```python
from build123d import *

# Parameters (mm, degrees)
F1_DEPTH  = 16
F2_W      = 70
F2_H      = 3
F3_DEPTH  = 2
F4_W      = 50
F4_H      = 14
F5_DEPTH  = 2
F6_R      = 1
F9_DEPTH  = 2
F11_DEPTH = 38.001
F13_D     = 4
F14_R     = 3
F14_R_2   = 2
F15_DEPTH = 5
F16_R     = 3


# Not quite as in the source:
# - a pattern or mirror of a feature is missing from the dataset's text; its kind, count and spacing are read off the source's solid


with BuildPart() as f1:
    # F0 (on Front) → F1 (new body)
    with BuildSketch(Plane.XZ):
        with BuildLine():
            Line((94, 11), (0, 11))
            ThreePointArc((0, 11), (-11, 0), (0, -11))
            Line((0, -11), (19, -11))
            ThreePointArc((19, -11), (21.7681124643, -11.8361612201), (23.6103896104, -14.064978646))
            ThreePointArc((23.6103896104, -14.064978646), (47.8977113224, -44.6078392712), (84.5520957277, -57.9942665386))
            ThreePointArc((84.5520957277, -57.9942665386), (89.5187953856, -59.3173941728), (93.6732506492, -62.3438233708))
            Line((93.6732506492, -62.3438233708), (95.1549842887, -61))
            ThreePointArc((95.1549842887, -61), (90.3976747979, -57.5207528796), (84.7034264019, -56))
            ThreePointArc((84.7034264019, -56), (49.0672193413, -42.9854179344), (25.4545454545, -13.2909701044))
            ThreePointArc((25.4545454545, -13.2909701044), (22.87535745, -10.1706257081), (19, -9))
            Line((19, -9), (0, -9))
            ThreePointArc((0, -9), (-9, 0), (0, 9))
            Line((0, 9), (94, 9))
            Line((94, 9), (94, 11))
        make_face()
    extrude(amount=F1_DEPTH)

    # F2 (on face) → F3 (join)
    with BuildSketch(Plane.XY.offset(11)):
        with Locations((59, -17.5)):
            Rectangle(F2_W, F2_H)
    extrude(amount=-F3_DEPTH)

    # F4 (on face) → F5 (join)
    with BuildSketch(Plane.XZ.offset(19)):
        with Locations((69, 2)):
            Rectangle(F4_W, F4_H)
    extrude(amount=-F5_DEPTH)

    # F6
    f6_edges = [f1.edges().sort_by_distance(p)[0] for p in [
        (59, -19, 11),
    ]]
    fillet(f6_edges, radius=F6_R)

    # F7: F1 across plane


with BuildPart() as f1_1:
    add(f1.part)
    add(f1.part.mirror(Plane.XZ))

    # F8 (on face) → F9 (cut)
    with BuildSketch(Plane.XY.offset(11)):
        with BuildLine():
            Line((94, 12), (34, 12))
            ThreePointArc((34, 12), (22, 0), (34, -12))
            Line((34, -12), (94, -12))
            Line((94, -12), (94, 12))
        make_face()
    extrude(amount=-F9_DEPTH, mode=Mode.SUBTRACT)

    # F10 (on face) → F11 (cut, through all)
    with BuildSketch(Plane.XZ.offset(19)):
        with BuildLine():
            ThreePointArc((50, 7.4429814443), (47, 4.4429814443), (50, 1.4429814443))
            Line((50, 1.4429814443), (70, 1.4429814443))
            ThreePointArc((70, 1.4429814443), (73, 4.4429814443), (70, 7.4429814443))
            Line((70, 7.4429814443), (50, 7.4429814443))
        make_face()
    extrude(amount=-F11_DEPTH, mode=Mode.SUBTRACT)

    # F13 (through all)
    with Locations(Plane.XZ.offset(19)):
        with Locations((80, 1)):
            Hole(F13_D / 2)

    # F14 (on face) → F15 (join)
    with BuildSketch(Plane(origin=(0, -17, 0), x_dir=(-1, 0, 0), z_dir=(0, 1, 0))):
        with Locations((-80, 1)):
            Circle(F14_R)
        with Locations((-80, 1)):
            Circle(F14_R_2, mode=Mode.SUBTRACT)
    f15 = extrude(amount=F15_DEPTH)

    # F15_copies: F15 across plane
    add(f15.mirror(Plane.ZX))

    # F16
    f16_edges = [f1_1.edges().sort_by_distance(p)[0] for p in [
        (94, 18, -5),
        (44, 18, -5),
        (94, -18, -5),
        (44, -18, -5),
    ]]
    fillet(f16_edges, radius=F16_R)


solid = f1_1.part
```
CAD build for the part. Positions are in the model's coordinates, mm. A direction names the side the tool comes from. Round coordinates to 2 decimals unless told otherwise and drop trailing zeros. Order: outer loops, then holes, each group sorted by start corner. A loop starts at its lowest first (then second) coordinate and runs counter-clockwise, first axis right, second up.
Q1. Two-plate mould, pull along X, no slides. Class faces 4 (the cylindrical face through (78.092, 15.549, 1.601)), 5 (the cylindrical face through (44.9, -17.99, -4.14)), 6 (the flat face through (9, 0, -11)): pulls with the +X half, pulls with the -X half, needs draft (parallel to the pull), parting line crosses it, or undercut.
Q2. Wall check: L1, parallel to Y at x = 91, z = -3; L2, parallel to Z at x = 80, y = 14.75; L3, parallel to Z at x = 13.5, y = 9.5. Give the ranges that are in metal, low to high.
Q3. Slice it at D-D (x = 80). State how many separate pieces and enclosed holes the cut face has, and give its area (3 significant figures).
Q4. Which spindle directions (+Z, -Z, +X, -X, +Y, -Y) get a long thin tool onto all of the face, cutting with end or side? Do faces 1 (the cylindrical face through (47, -18, 4.5)), 2 (the cylindrical face through (83, -15, 1)), 3 (the cylindrical face through (22.92, -0.22, -10.2)). Say none if no direction does.
Q5. Drop flat-ended pins along their axis: pin 1 (5 mm diameter, centred on x = 50, z = -43.5, fed in from +Y); pin 2 (1.6 mm diameter, centred on x = 59, y = 17.5, fed in from -Z); pin 3 (3 mm diameter, centred on y = 7.5, z = -30, fed in from +X); pin 4 (1 mm diameter, centred on x = 62.5, y = -18.5, fed in from +Z). Give the stop position or say it passes through.
Q6. Slice it at A-A (y = -14.5). Write the cut outline in (x, z).
Q7. Slice it at C-C (x = 28). Write the cut outline in (y, z).
Q8. Slice it at B-B (x = 6). Write the cut outline in (y, z), and give its area (3 significant figures).
Results below:
1. face 4: undercut
1. face 5: pulls with the -X half
1. face 6: needs draft
2. L1: y = -19 to -17, 17 to 19
2. L2: z = -57.5 to -55.48, -2 to -1, 3 to 4, 9 to 11
2. L3: z = -11 to -9, 9 to 11
3. separate pieces: 5
3. enclosed holes: 0
3. area: 152 mm2
4. face 1: +Y, -Y
4. face 2: none
4. face 3: +X, +Y, -Y
5. pin 1: stops at y = 16
5. pin 2: stops at z = -5
5. pin 3: stops at x = 36.63
5. pin 4: stops at z = 11
6. outline: (0, -11) - (19, -11) arc R5 cw to (23.61, -14.06) arc R72 ccw to (84.55, -57.99) arc R14 cw to (93.67, -62.34) - (95.15, -61) arc R16 ccw to (84.7, -56) arc R70 cw to (25.45, -13.29) arc R7 ccw to (19, -9) - (0, -9) arc R9 cw to (0, 9) - (94, 9) - (94, 11) - (0, 11) arc R11 ccw to start; circle Ø6 at (80, 1); hole circle Ø4 at (80, 1)
7. outline: (-19, 9) - (-10.39, 9) - (-10.39, 11) - (-18, 11) arc R1 ccw to (-19, 10) - close; (-16, -22.81) - (16, -22.81) - (16, -18.7) - (-16, -18.7) - close; (10.39, 9) - (19, 9) - (19, 10) arc R1 ccw to (18, 11) - (10.39, 11) - close
8. outline: (-16, -11) - (16, -11) - (16, -9) - (-16, -9) - close; (-16, 9) - (16, 9) - (16, 11) - (-16, 11) - close
8. area: 128 mm2
